Verification items for the finished model (mm, model axes). Face numbers are marked on the shaded views. A direction names the side the tool comes from. Round coordinates to 2 decimals unless told otherwise and drop trailing zeros. Write each loop counter-clockwise with the first axis right and the second up, starting at its lowest first coordinate (ties: lowest second). Pieces come first, ordered by that corner, then holes. Notation, with made-up numbers: (86.5, 7.5) - (139.5, 7.5) arc R19 ccw to (139.5, 18.5) - close; hole circle Ø1 at (26, 27.25). An arc over 180 degrees is marked (long way). Answer as a JSON object with one key per item and string values. Group by question number.
1) Set-up check for the marked faces 4, 5, 6 and 7: record each of +Z, -Z, +X, -X, +Y, -Y from which the full face is reachable in a straight line by a thin tool's end or side.
2) Section check A-A (x = 9.5). Enter the section's corners in (y, z).
3) Thickness scan on line 1 (X direction, y = 0, z = 1.25); line 2 (X direction, y = 9.5, z = 13.25); line 3 (Z direction, x = -2, y = 12). Record the ranges inside material, lowest first.
4) Section check C-C (z = 4). Enter the section's corners in (x, y).
5) Section check D-D (y = 7.5). Enter the section's corners in (x, z), then the cut area to 3 significant figures.
6) Mould release check, pull along Y, two halves, no side actions. Record for the marked faces 1, 2 and 3: +Y half, -Y half, draft (parallel to the pull), parting line (faces both ways), or undercut.
7) Go/stop test with flat-tipped pins: pin 1 Ø8 at (y, z) = (5, 12.5) entering from +X; pin 2 Ø1.6 at (x, y) = (20.5, -1.5) entering from +Z; pin 3 Ø2.5 at (x, y) = (-20, 5.5) entering from +Z; pin 4 Ø8 at (x, z) = (12, 19.5) entering from +Y. Record where each tip stops, or that it passes through.
8) Section check B-B (y = 0). Enter the section's corners in (x, z), then the cut area to 3 significant figures.
Autodesk Inventor part; units mm, degrees
ref_plane "YZ Plane" through (0, 0, 0) normal (1, 0, 0) x (0, 1, 0)
ref_plane "XZ Plane" through (0, 0, 0) normal (0, 1, 0) x (-1, 0, 0)
ref_plane "XY Plane" through (0, 0, 0) normal (0, 0, 1) x (1, 0, 0)
sketch "Skizze1" plane through (0, 0, 0) normal (0, 0, 1) x (1, 0, 0)
  line L0 (-25, -14) -> (25, -14)
  line L1 (25, -14) -> (25, 14)
  line L2 (25, 14) -> (-25, 14)
  line L3 (-25, 14) -> (-25, -14)
  line L4 (-25, -14) -> (25, 14) construction
  line L5 (25, -14) -> (-25, 14) construction
  line L6 (-13.5, -10) -> (13.5, -10)
  line L7 (13.5, -10) -> (13.5, 10)
  line L8 (13.5, 10) -> (-13.5, 10)
  line L9 (-13.5, 10) -> (-13.5, -10)
  line L10 (-13.5, -10) -> (13.5, 10) construction
  line L11 (13.5, -10) -> (-13.5, 10) construction
  circle A0 centre (-20.5, 0) radius 1.75
  circle A1 centre (20.5, 0) radius 1.75
  line L12 (-20.5, 0) -> (20.5, 0) construction
  point P0 (0, 0)
  point P1 (0, 0)
  point P2 (0, 0)
  point P3 (0, 0)
  dimension "d0" = 50
  dimension "d1" = 20
  dimension "d2" = 27
  dimension "d3" = 41
  dimension "d4" = 3.5
  dimension "d5" = 28
extrude "Extrusion1" add sketch "Skizze1" along normal blind 6
sketch "Skizze2" plane through (0, 0, 6) normal (0, 0, 1) x (1, 0, 0)
  line L0 (-13.5, -10) -> (-13.5, 10)
  line L1 (-13.5, 10) -> (13.5, 10)
  line L2 (13.5, 10) -> (13.5, -10)
  line L3 (13.5, -10) -> (-13.5, -10)
  circle A0 centre (20.5, 0) radius 1.75
  circle A1 centre (-20.5, 0) radius 1.75
  line L4 (-25, -14) -> (25, -14)
  line L5 (25, -14) -> (25, 14)
  line L6 (25, 14) -> (-25, 14)
  line L7 (-25, 14) -> (-25, -14)
  line L8 (-20.5, 3.1754) -> (-17.75, 1.5877)
  line L9 (-17.75, 1.5877) -> (-17.75, -1.5877)
  line L10 (-17.75, -1.5877) -> (-20.5, -3.1754)
  line L11 (-20.5, -3.1754) -> (-23.25, -1.5877)
  line L12 (-23.25, -1.5877) -> (-23.25, 1.5877)
  line L13 (-23.25, 1.5877) -> (-20.5, 3.1754)
  line L14 (20.5, 3.1754) -> (23.25, 1.5877)
  line L15 (23.25, 1.5877) -> (23.25, -1.5877)
  line L16 (23.25, -1.5877) -> (20.5, -3.1754)
  line L17 (20.5, -3.1754) -> (17.75, -1.5877)
  line L18 (17.75, -1.5877) -> (17.75, 1.5877)
  line L19 (17.75, 1.5877) -> (20.5, 3.1754)
  line L20 (-25, 14) -> (-25, -14)
  line L21 (25, -14) -> (25, 14)
  point P0 (0, 0)
  dimension "d8" = 5.5
extrude "Extrusion2" cut sketch "Skizze2" against normal blind 3 contours A0 | A1 | L8 L9 L10 L11 L12 L13 | L14 L15 L16 L17 L18 L19
sketch "Skizze3" plane through (0, 0, 6) normal (0, 0, 1) x (1, 0, 0)
  line L0 (-23.25, 1.5877) -> (-20.5, 3.1754)
  line L1 (-20.5, 3.1754) -> (-17.75, 1.5877)
  line L2 (-17.75, 1.5877) -> (-17.75, -1.5877)
  line L3 (-17.75, -1.5877) -> (-20.5, -3.1754)
  line L4 (-20.5, -3.1754) -> (-23.25, -1.5877)
  line L5 (-23.25, -1.5877) -> (-23.25, 1.5877)
  line L6 (17.75, 1.5877) -> (20.5, 3.1754)
  line L7 (20.5, 3.1754) -> (23.25, 1.5877)
  line L8 (23.25, 1.5877) -> (23.25, -1.5877)
  line L9 (23.25, -1.5877) -> (20.5, -3.1754)
  line L10 (20.5, -3.1754) -> (17.75, -1.5877)
  line L11 (17.75, -1.5877) -> (17.75, 1.5877)
  line L12 (-13.5, -10) -> (-13.5, 10)
  line L13 (-13.5, 10) -> (13.5, 10)
  line L14 (13.5, 10) -> (13.5, -10)
  line L15 (13.5, -10) -> (-13.5, -10)
  line L16 (-25, -14) -> (25, -14)
  line L17 (25, -14) -> (25, 14)
  line L18 (25, 14) -> (-25, 14)
  line L19 (-25, 14) -> (-25, -14)
  line L20 (-16.5, -14) -> (16.5, -14)
  line L21 (16.5, -14) -> (16.5, 14)
  line L22 (16.5, 14) -> (-16.5, 14)
  line L23 (-16.5, 14) -> (-16.5, -14)
  line L24 (-16.5, -14) -> (16.5, 14) construction
  line L25 (16.5, -14) -> (-16.5, 14) construction
  point P0 (0, 0)
  dimension "d11" = 3
extrude "Extrusion3" add sketch "Skizze3" along normal blind 14 contours L23 L18 L21 L16
sketch "Skizze4" plane through (0, 0, 20) normal (0, 0, 1) x (1, 0, 0)
  line L0 (-13.5, 10) -> (13.5, 10)
  line L1 (13.5, 10) -> (13.5, -10)
  line L2 (13.5, -10) -> (-13.5, -10)
  line L3 (-13.5, -10) -> (-13.5, 10)
  line L4 (16.5, 14) -> (-16.5, 14)
  line L5 (-16.5, 14) -> (-16.5, -14)
  line L6 (-16.5, -14) -> (16.5, -14)
  line L7 (16.5, -14) -> (16.5, 14)
  point P0 (0, 0)
extrude "Extrusion4" add sketch "Skizze4" along normal blind 2 contours L0 L1 L2 L3 | L7 L6 L5 L4
sketch "Skizze5" plane through (-13.5, 10, 0) normal (0, -1, 0) x (1, 0, 0)
  line L0 (27, 0) -> (0, 0)
  line L1 (27, 0) -> (27, 20)
  line L2 (0, 20) -> (27, 20)
  line L3 (0, 0) -> (0, 20)
  line L4 (38.5, 0) -> (-11.5, 0)
  line L5 (-11.5, 0) -> (-11.5, 6)
  line L6 (-3, 6) -> (-11.5, 6)
  line L7 (-3, 6) -> (-3, 22)
  line L8 (30, 22) -> (-3, 22)
  line L9 (30, 6) -> (30, 22)
  line L10 (38.5, 6) -> (30, 6)
  line L11 (38.5, 0) -> (38.5, 6)
  line L12 (0, 6) -> (27, 6)
  line L13 (27, 6) -> (27, 20)
  line L14 (27, 20) -> (0, 20)
  line L15 (0, 20) -> (0, 6)
  line L16 (0, 6) -> (27, 20) construction
  line L17 (27, 6) -> (0, 20) construction
  point P0 (13.5, 0)
  point P1 (13.5, 13)
extrude "Extrusion5" cut sketch "Skizze5" against normal through all contours L12 L3 L2 L1
sketch "Skizze7" plane through (-25, 14, 0) normal (0, 1, 0) x (1, 0, 0)
  line L0 (38.5, 0) -> (38.5, -6)
  line L1 (11.5, -20) -> (11.5, -6)
  line L2 (11.5, -6) -> (38.5, -6)
  line L3 (38.5, -6) -> (38.5, -20)
  line L4 (38.5, -20) -> (11.5, -20)
  line L5 (50, 0) -> (0, 0)
  line L6 (0, 0) -> (0, -6)
  line L7 (8.5, -6) -> (0, -6)
  line L8 (8.5, -6) -> (8.5, -22)
  line L9 (41.5, -22) -> (8.5, -22)
  line L10 (41.5, -6) -> (41.5, -22)
  line L11 (50, -6) -> (41.5, -6)
  line L12 (50, 0) -> (50, -6)
  point P0 (25, 0)
extrude "Extrusion6" add sketch "Skizze7" along normal blind 6
chamfer "Fase1" distance 5 angle 45 1 edges at (0, 10, 6)
fillet "Rundung1" radius 8 4 edges at (25, -14, 3) (25, 20, 3) (-25, -14, 3) (-25, 20, 3)
properties part number "kaltgeraete"
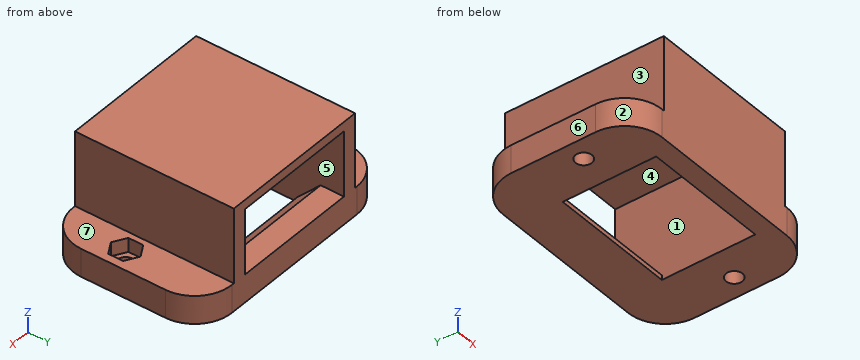
Returned:
{
 "1": {"face 4": "+Y", "face 5": "none", "face 6": "+Z, -Z, -X, +Y, -Y", "face 7": "+Z, +X, +Y, -Y"},
 "2": {"outline": "(-14, 0) - (-10, 0) - (-10, 20) - (20, 20) - (20, 22) - (-14, 22) - close; (10, 0) - (20, 0) - (20, 6) - (15, 6) - (10, 1) - close"},
 "3": {"line 1": "-25 to -22.25, -18.75 to -13.5, 13.5 to 18.75, 22.25 to 25", "line 2": "-16.5 to -13.5, 13.5 to 16.5", "line 3": "0 to 3, 20 to 22"},
 "4": {"outline": "(-25, -6) arc R8 ccw to (-17, -14) - (17, -14) arc R8 ccw to (25, -6) - (25, 12) arc R8 ccw to (17, 20) - (-17, 20) arc R8 ccw to (-25, 12) - close; hole (-23.25, -1.59) - (-20.5, -3.18) - (-17.75, -1.59) - (-17.75, 1.59) - (-20.5, 3.18) - (-23.25, 1.59) - close; hole (-13.5, -10) - (13.5, -10) - (13.5, 13) - (-13.5, 13) - close; hole (17.75, -1.59) - (20.5, -3.18) - (23.25, -1.59) - (23.25, 1.59) - (20.5, 3.18) - (17.75, 1.59) - close"},
 "5": {"outline": "(-25, 0) - (-13.5, 0) - (-13.5, 20) - (13.5, 20) - (13.5, 0) - (25, 0) - (25, 6) - (16.5, 6) - (16.5, 22) - (-16.5, 22) - (-16.5, 6) - (-25, 6) - close", "area": "288 mm2"},
 "6": {"face 1": "undercut", "face 2": "-Y half", "face 3": "draft"},
 "7": {"pin 1": "x = 16.5", "pin 2": "z = 3", "pin 3": "z = 6", "pin 4": "y = 20"},
 "8": {"outline": "(-25, 0) - (-22.25, 0) - (-22.25, 3) - (-23.25, 3) - (-23.25, 6) - (-25, 6) - close; (-18.75, 0) - (-13.5, 0) - (-13.5, 20) - (13.5, 20) - (13.5, 0) - (18.75, 0) - (18.75, 3) - (17.75, 3) - (17.75, 6) - (16.5, 6) - (16.5, 22) - (-16.5, 22) - (-16.5, 6) - (-17.75, 6) - (-17.75, 3) - (-18.75, 3) - close; (22.25, 0) - (25, 0) - (25, 6) - (23.25, 6) - (23.25, 3) - (22.25, 3) - close", "area": "234 mm2"}
}
